Read the model definition and answer for the solid it produces. Units are mm, in the model's axes. Give positions to 0.01 mm unless a question says otherwise; leave off trailing zeros. Write each loop counter-clockwise with the first axis right and the second up, starting at its lowest first coordinate (ties: lowest second). Pieces come first, ordered by that corner, then holes. Notation, with made-up numbers: (-28.5, 40.5) - (-11.5, 40.5) arc R28 ccw to (-11.5, 69.5) - close; hole circle Ø4 at (40.25, -1). An arc over 180 degrees is marked (long way). Answer as a JSON object with one key per item and string values. Group by question number.
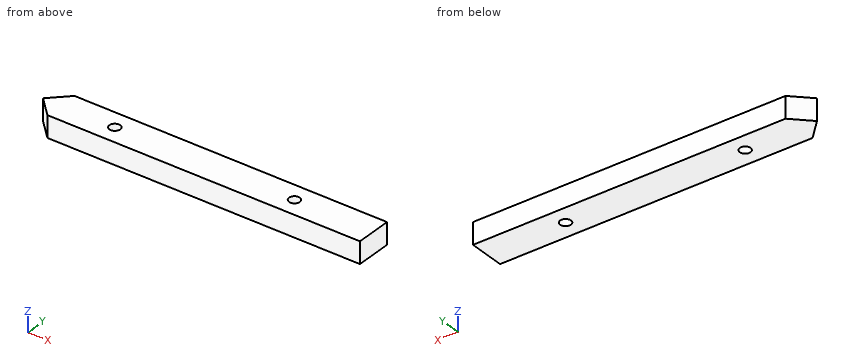
```python
from build123d import *

# Parameters (mm, degrees)
ESQUISSE1_W             = 92
ESQUISSE1_H             = 10
BOSS_EXTRU_1_DEPTH      = 6
ENL_V_MAT_EXTRU_1_DEPTH = 6
ENL_V_MAT_EXTRU_2_DEPTH = 6
ESQUISSE4_R             = 1.5
ENL_V_MAT_EXTRU_3_DEPTH = 6


with BuildPart() as part:
    # Esquisse1 → Boss.-Extru.1 (new body)
    with BuildSketch(Plane.XY):
        Rectangle(ESQUISSE1_W, ESQUISSE1_H)
    extrude(amount=BOSS_EXTRU_1_DEPTH)

    # Esquisse2 → Enlèv. mat.-Extru.1 (cut)
    with BuildSketch(Plane.XY.offset(6)):
        Polygon((-46, -5), (-46, 0), (-41, -5), align=None)
    extrude(amount=-ENL_V_MAT_EXTRU_1_DEPTH, mode=Mode.SUBTRACT)

    # Esquisse3 → Enlèv. mat.-Extru.2 (cut)
    with BuildSketch(Plane.XY.offset(6)):
        Polygon((-46, 0), (-41, 5), (-46, 5), align=None)
    extrude(amount=-ENL_V_MAT_EXTRU_2_DEPTH, mode=Mode.SUBTRACT)

    # Esquisse4 → Enlèv. mat.-Extru.3 (cut)
    with BuildSketch(Plane.XY.offset(6)):
        with Locations((-26, 0)):
            Circle(ESQUISSE4_R)
        with Locations((24, 0)):
            Circle(ESQUISSE4_R)
    extrude(amount=-ENL_V_MAT_EXTRU_3_DEPTH, mode=Mode.SUBTRACT)


solid = part.part
```
1) Find section A-A, the plane z = 4.9. Write down the section's boundary in (x, y).
2) Find section B-B, the plane x = 24. Write down the section's boundary in (y, z), and give its area (3 significant figures).
3) Find the intervals of material crossed by line 1 (X direction, y = 0.25, z = 3.1); line 2 (Y direction, x = -26, z = 4.1); line 3 (X direction, y = 2.25, z = 3.4), in increasing order. Write a range as [from, to].
Values follow:
{
 "1": {"outline": "(-46, 0) - (-41, -5) - (46, -5) - (46, 5) - (-41, 5) - close; hole circle Ø3 at (-26, 0); hole circle Ø3 at (24, 0)"},
 "2": {"outline": "(-5, 0) - (-1.5, 0) - (-1.5, 6) - (-5, 6) - close; (1.5, 0) - (5, 0) - (5, 6) - (1.5, 6) - close", "area": "42.0 mm2"},
 "3": {"line 1": "x = [-45.75, -27.48], [-24.52, 22.52], [25.48, 46]", "line 2": "y = [-5, -1.5], [1.5, 5]", "line 3": "x = [-43.75, 46]"}
}
